Could you check a few things on this model? Use its own coordinates, in mm. Face numbers are marked on the shaded views. A direction names the side the tool comes from. Round coordinates to 2 decimals unless told otherwise and drop trailing zeros. Loops run counter-clockwise (first coordinate to the right, second up) from the corner with the lowest first, then second, coordinate; pieces in that order, holes last. Notation, with made-up numbers: (-5, 76.25) -> (25, 76.25) arc R16 ccw to (25, 80.25) -> close; hole circle Ø10 at (-38.75, -22.75). An arc over 180 degrees is marked (long way). Write each question's results on one line, items separated by ' | '. Start each with the question number.
1) Imagine slicing it at A-A, the plane x = 0. Give the number of separate pieces and of enclosed holes in the cut face, plus the area to 3 significant figures.
2) Which directions (+Z, -Z, +X, -X, +Y, -Y) give clear straight access to the entire face, cutting with the end or side of a thin tool? Please do the marked faces 4 and 5.
3) If I drill on probe 1 along X at (y, z) = (7.5, 0); probe 2 along Y at (x, z) = (-5.5, -4.75); probe 3 along Z at (x, y) = (8, 2.55), over which ranges is the centre line in solid material (lowest first)?
4) Imagine slicing it at B-B, the plane y = 7. List the corners of the cut face in (x, z) for me.
5) For P1, Ø6, axis at x = 3.5, y = 13, coming from the -Z side; P2, Ø4, axis at x = 0, z = -8, coming from the +Y side; P3, Ø12, axis at x = 3.5, z = 5, coming from the +Y side; P4, Ø2, axis at x = -2, y = 5.5, coming from the -Z side, each with a flat end and sliding along its axis, tell me the tip position at first contact or that it passes through.
6) We'd pull the mould along X, two halves only. Please class the marked faces 1, 2 and 3: pulls with the +X half, pulls with the -X half, needs draft (parallel to the pull), parting line crosses it, or undercut.
from build123d import *

# Parameters (mm, degrees)
CUT_EXTRUDE1_DEPTH       = 22.610182785
CUT_EXTRUDE1_DEPTH_BACK  = 22.610182785
SKETCH2_R                = 4
M3_CLEARANCE_HOLE1_D     = 3.4
M3_CLEARANCE_HOLE1_DEPTH = 10
M3_CLEARANCE_HOLE1_TIP   = 1.021463052
CHAMFER1_SIZE            = 0.25


with BuildPart() as part:
    # Sketch1 → Revolve1 (revolve)
    with BuildSketch(Plane.XY, mode=Mode.PRIVATE) as revolve1_sk:
        Polygon((0, 0), (5.1, 0), (5.1, 1.5), (11, 1.5), (11, 5), (5.1, 5), (5.1, 15), (0, 15), align=None)
    revolve(revolve1_sk.sketch.rotate(Axis((0, 0, 0), (0, -1, 0)), 90), axis=Axis((0, 0, 0), (0, -1, 0)))

    # Sketch2 → Cut-Extrude1 (cut, two sides: drawn at the far end of the back side and taken through both)
    with BuildSketch(Plane.XZ.offset(-CUT_EXTRUDE1_DEPTH_BACK)):
        with Locations(Location((0, 0, 0), (0, 0, 270))):
            Circle(SKETCH2_R)
    extrude(amount=CUT_EXTRUDE1_DEPTH + CUT_EXTRUDE1_DEPTH_BACK, mode=Mode.SUBTRACT)

    # M3 Clearance Hole1
    with Locations(Plane.XZ.offset(-1.5)):
        with Locations((0, 8), (8, 0), (0, -8), (-8, 0), (0, 0)):
            Hole(M3_CLEARANCE_HOLE1_D / 2, depth=M3_CLEARANCE_HOLE1_DEPTH)
            with Locations((0, 0, -(M3_CLEARANCE_HOLE1_DEPTH + M3_CLEARANCE_HOLE1_TIP / 2))):  # 118° drill point
                Cone(0, M3_CLEARANCE_HOLE1_D / 2, M3_CLEARANCE_HOLE1_TIP, mode=Mode.SUBTRACT)

    # Chamfer1
    chamfer1_edges = [part.edges().sort_by_distance(p)[0] for p in [
        (0, 15, 4),
        (0, 15, -5.1),
        (0, 5, -5.1),
        (0, 5, -11),
        (0, 1.5, -11),
        (0, 1.5, -5.1),
        (0, 0, -5.1),
    ]]
    chamfer(chamfer1_edges, length=CHAMFER1_SIZE)


solid = part.part
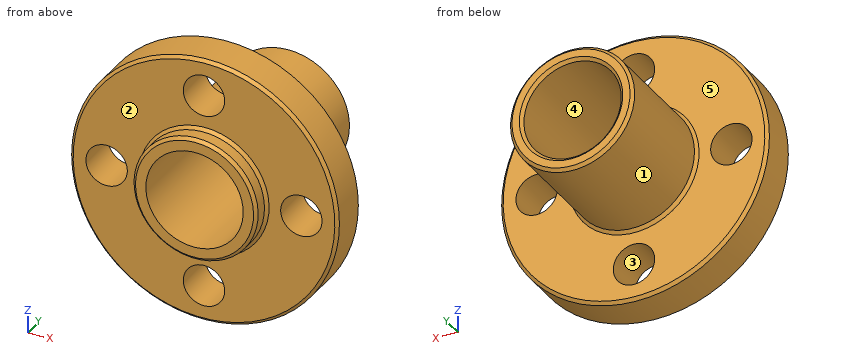
Checked values:
1) separate pieces: 4 | enclosed holes: 0 | area: 50.3 mm^2
2) face 4: +Y, -Y | face 5: +Y
3) probe 1: -5.1 to -4, 4 to 5.1 | probe 2: 1.5 to 5 | probe 3: -7.55 to -1.7, 1.7 to 7.55
4) outline: circle Ø10.2 at (0, 0); hole circle Ø8 at (0, 0)
5) P1: z = -5.08 | P2: y = 5 | P3: y = 15 | P4: z = -10.92
6) face 1: parting line crosses it | face 2: needs draft | face 3: undercut
